Solid Edge part; units mm, degrees
sketch "Sketch1" plane through (0, 0, 0) normal (1, 0, 0) x (0, 1, 0)
  line L0 (219.0526, 30.5) -> (-2.5, 30.5)
  arc A0 (-2.5, 30.5) -> (-6.8265, 29.2292) centre (-2.5, 22.5) ccw
  line L1 (-6.8265, 29.2292) -> (-29.379, 14.7292)
  arc A1 (-29.379, 14.7292) -> (-21.0939, 1.0481) centre (-25.0526, 8) ccw
  line L2 (-21.0939, 1.0481) -> (7.5259, 17.345)
  arc A2 (7.5259, 17.345) -> (10, 18) centre (10, 13) cw
  line L3 (10, 18) -> (207.0526, 18)
  arc A3 (207.0526, 18) -> (208.7444, 17.7051) centre (207.0526, 13) cw
  line L4 (208.7444, 17.7051) -> (216.3457, 14.9719)
  arc A4 (216.3457, 14.9719) -> (219.0526, 30.5) centre (219.0526, 22.5) ccw
  line L5 (219.0526, 27.5) -> (-2.5, 27.5)
  arc A5 (-2.5, 27.5) -> (-5.204, 26.7057) centre (-2.5, 22.5) ccw
  line L6 (-5.204, 26.7057) -> (-27.7566, 12.2057)
  arc A6 (-27.7566, 12.2057) -> (-22.5784, 3.655) centre (-25.0526, 8) ccw
  line L7 (-22.5784, 3.655) -> (6.0414, 19.9519)
  arc A7 (6.0414, 19.9519) -> (10, 21) centre (10, 13) cw
  line L8 (10, 21) -> (207.0526, 21)
  arc A8 (207.0526, 21) -> (209.7595, 20.5281) centre (207.0526, 13) cw
  line L9 (209.7595, 20.5281) -> (217.3607, 17.7949)
  arc A9 (217.3607, 17.7949) -> (219.0526, 27.5) centre (219.0526, 22.5) ccw
extrude "Protrusion1" add sketch "Sketch1" along normal blind 4
properties material "Steel"
Can you work these out from the model? Positions are in its coordinate system, mm. A direction names the side the tool comes from. Coordinates: 2 decimals unless noted, no trailing zeros. Loops run counter-clockwise (first coordinate to the right, second up) from the corner with the lowest first, then second, coordinate; pieces in that order, holes last. Notation, with made-up numbers: (-39, 8) -> (10, 8) arc R27 cw to (10, 46) -> close; hole circle Ø1 at (45, 50). An arc over 180 degrees is marked (long way). Answer as a JSON object with one key per item and string values.
1) For faces 1 (the face through (4, 86.8, 20.8)), 2 (the face through (2, 107, 18)), 3 (the face through (1.97, -16.32, 19.56)), which set-ups out of +Z, -Z, +X, -X, +Y, -Y let a thin tool reach every point of the face, with its end or its side?
Results:
{"face 1": "+Z, -Z, +X, +Y, -Y", "face 2": "-Z, +X, -X", "face 3": "+X, -X"}
2) Imagine slicing it at A-A (y = 19). Please give me the cut outline in (x, z), then the cut area to 3 significant figures.
Results:
{"outline": "(0, 18) -> (4, 18) -> (4, 21) -> (0, 21) -> close; (0, 27.5) -> (4, 27.5) -> (4, 30.5) -> (0, 30.5) -> close", "area": "24.0 mm^2"}
3) Imagine slicing it at B-B (z = 8). Please give me the cut outline in (x, y).
Results:
{"outline": "(0, -33.05) -> (4, -33.05) -> (4, -30.05) -> (0, -30.05) -> close; (0, -14.95) -> (4, -14.95) -> (4, -8.89) -> (0, -8.89) -> close"}
4) Imagine slicing it at C-C (x = 3.1). Please give me the cut outline in (y, z).
Results:
{"outline": "(-29.38, 14.73) arc R8 ccw to (-21.09, 1.05) -> (7.53, 17.34) arc R5 cw to (10, 18) -> (207.05, 18) arc R5 cw to (208.74, 17.71) -> (216.35, 14.97) arc R8 ccw (long way) to (219.05, 30.5) -> (-2.5, 30.5) arc R8 ccw to (-6.83, 29.23) -> close; hole (-27.76, 12.21) arc R5 ccw to (-22.58, 3.66) -> (6.04, 19.95) arc R8 cw to (10, 21) -> (207.05, 21) arc R8 cw to (209.76, 20.53) -> (217.36, 17.79) arc R5 ccw (long way) to (219.05, 27.5) -> (-2.5, 27.5) arc R5 ccw to (-5.2, 26.71) -> close"}
5) If I drill on line 1 (Z direction, x = 1.4, y = 89); line 2 (Y direction, x = 1.15, z = 22.5); line 3 (Y direction, x = 2.75, z = 25), over which ranges is the centre line in solid material (lowest first)?
Results:
{"line 1": "z = 18 to 21, 27.5 to 30.5", "line 2": "y = -17.29 to -11.75, 224.05 to 227.05", "line 3": "y = -13.4 to -7.86, 223.38 to 226.65"}
6) For P1, Ø1.5, axis at x = 1, y = 161.5, coming from the -Z side, with a flat end and sliding along its axis, tell me the tip position at first contact or that it passes through.
Results:
{"P1": "stops at z = 18"}
7) Thinking about a two-plate mould opening in Y: for faces 4 (the face through (1.97, 212.49, 16.36)), 5 (the face through (2, -31.8, 3.7)), 6 (the face through (1.972, -4.785, 30.167)), which applies, pulls with the +Y half, pulls with the -Y half, needs draft (parallel to the pull), parting line crosses it, or undercut?
Results:
{"face 4": "undercut", "face 5": "parting line crosses it", "face 6": "pulls with the -Y half"}
